```python
from build123d import *

# Parameters (mm, degrees)
SKETCH1_R           = 2.75
BOSS_EXTRUDE1_DEPTH = 6
FILLET1_R           = 3
SKETCH2_R           = 25.25
CUT_EXTRUDE1_DEPTH  = 3


with BuildPart() as part:
    # Sketch1 → Boss-Extrude1 (new body)
    with BuildSketch(Plane(origin=(0, 0, 0), x_dir=(1, 0, 0), z_dir=(0, 1, 0))):
        with BuildLine():
            Line((-57.629202667, 39.951533137), (-39.951533137, 57.629202667))
            Line((-39.951533137, 57.629202667), (-21.213203436, 38.890872965))
            ThreePointArc((-21.213203436, 38.890872965), (0, 30.104076401), (21.213203436, 38.890872965))
            Line((21.213203436, 38.890872965), (39.951533137, 57.629202667))
            Line((39.951533137, 57.629202667), (57.629202667, 39.951533137))
            Line((57.629202667, 39.951533137), (35.355339059, 17.67766953))
            Line((35.355339059, 17.67766953), (35.355339059, -17.67766953))
            Line((35.355339059, -17.67766953), (57.629202667, -39.951533137))
            Line((57.629202667, -39.951533137), (39.951533137, -57.629202667))
            Line((39.951533137, -57.629202667), (21.213203436, -38.890872965))
            ThreePointArc((21.213203436, -38.890872965), (0, -30.104076401), (-21.213203436, -38.890872965))
            Line((-21.213203436, -38.890872965), (-39.951533137, -57.629202667))
            Line((-39.951533137, -57.629202667), (-57.629202667, -39.951533137))
            Line((-57.629202667, -39.951533137), (-35.355339059, -17.67766953))
            Line((-35.355339059, -17.67766953), (-35.355339059, 17.67766953))
            Line((-35.355339059, 17.67766953), (-57.629202667, 39.951533137))
        make_face()
        with Locations(Location((-45.254833996, 45.254833996, 0), (0, 0, 270))):
            Circle(SKETCH1_R, mode=Mode.SUBTRACT)
        with Locations(Location((45.254833996, 45.254833996, 0), (0, 0, 270))):
            Circle(SKETCH1_R, mode=Mode.SUBTRACT)
        with Locations(Location((45.254833996, -45.254833996, 0), (0, 0, 270))):
            Circle(SKETCH1_R, mode=Mode.SUBTRACT)
        with Locations(Location((-45.254833996, -45.254833996, 0), (0, 0, 270))):
            Circle(SKETCH1_R, mode=Mode.SUBTRACT)
        with Locations(Location((-24.75, 24.75, 0), (0, 0, 270))):
            Circle(SKETCH1_R, mode=Mode.SUBTRACT)
        with Locations(Location((-24.75, -24.75, 0), (0, 0, 270))):
            Circle(SKETCH1_R, mode=Mode.SUBTRACT)
        with Locations(Location((24.75, -24.75, 0), (0, 0, 90))):
            Circle(SKETCH1_R, mode=Mode.SUBTRACT)
        with Locations(Location((24.75, 24.75, 0), (0, 0, 90))):
            Circle(SKETCH1_R, mode=Mode.SUBTRACT)
        with Locations(Location((-14.142135624, 14.142135624, 0), (0, 0, 270))):
            Circle(SKETCH1_R, mode=Mode.SUBTRACT)
        with Locations(Location((14.142135624, 14.142135624, 0), (0, 0, 270))):
            Circle(SKETCH1_R, mode=Mode.SUBTRACT)
        with Locations(Location((14.142135624, -14.142135624, 0), (0, 0, 270))):
            Circle(SKETCH1_R, mode=Mode.SUBTRACT)
        with Locations(Location((-14.142135624, -14.142135624, 0), (0, 0, 270))):
            Circle(SKETCH1_R, mode=Mode.SUBTRACT)
    extrude(amount=BOSS_EXTRUDE1_DEPTH)

    # Fillet1
    fillet1_edges = [part.edges().sort_by_distance(p)[0] for p in [
        (-57.629202667, 3, -39.951533137),
        (-39.951533137, 3, -57.629202667),
        (39.951533137, 3, -57.629202667),
        (57.629202667, 3, -39.951533137),
        (57.629202667, 3, 39.951533137),
        (39.951533137, 3, 57.629202667),
        (-39.951533137, 3, 57.629202667),
        (-57.629202667, 3, 39.951533137),
    ]]
    fillet(fillet1_edges, radius=FILLET1_R)

    # Sketch2 → Cut-Extrude1 (cut)
    with BuildSketch(Plane(origin=(0, 6, 0), x_dir=(1, 0, 0), z_dir=(0, 1, 0))):
        with Locations(Location((0, 0, 0), (0, 0, 270))):
            Circle(SKETCH2_R)
    extrude(amount=-CUT_EXTRUDE1_DEPTH, mode=Mode.SUBTRACT)


solid = part.part
```
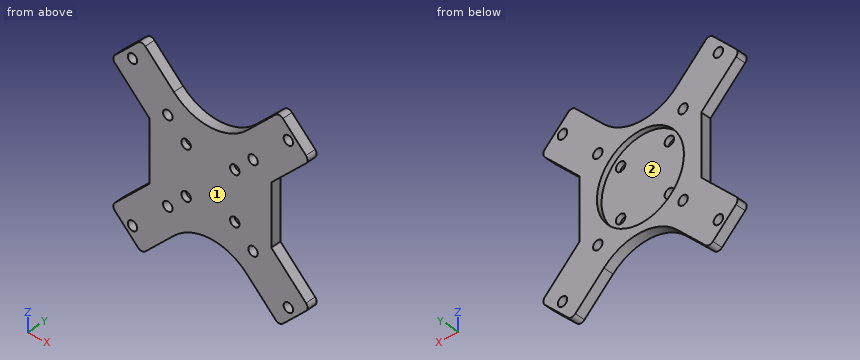
Check sheet for the modelled part. Datum: model origin and axes. Units: mm. Face numbers are marked on the shaded views. Coordinates: 2 decimals unless noted, no trailing zeros. Loops run counter-clockwise (first coordinate to the right, second up) from the corner with the lowest first, then second, coordinate; pieces in that order, holes last.
1) Sectioned sample at C-C (y = 4.15). Count the separate pieces of the cut face and the enclosed holes in it, and give its area (3 significant figures).
2) Sectioned sample at B-B (x = 0). Record the boundary of the cut face in (y, z).
3) Sectioned sample at D-D (z = -15). Record the boundary of the cut face in (x, y), and give its area (3 significant figures).
4) Release check for a two-part mould opening along X. For the marked faces 1 and 2 record: released by +X, released by -X, zero draft, split by the parting line, or undercut.
5) Material ranges on probe 1 along X at (y, z) = (4.95, -45); probe 2 along Z at (x, y) = (25.5, 4.5), recorded low to high.
6) Gauge pin test, flat ends, axial feed: pin 1 (1.8 mm diameter, centred on y = 1.5, z = 4, fed in from -X); pin 2 (4.5 mm diameter, centred on x = 14.14, z = 14.14, fed in from +Y); pin 3 (1.5 mm diameter, centred on x = -0.5, y = 1.5, fed in from +Z). Record the tip position at first contact, or that the pin passes through.
7) Sectioned sample at A-A (z = 0). Record the boundary of the cut face in (x, y).
Check sheet entries:
1. separate pieces: 1
1. enclosed holes: 9
1. area: 5,080 mm2
2. outline: (0, -30.1) - (6, -30.1) - (6, -25.25) - (3, -25.25) - (3, 25.25) - (6, 25.25) - (6, 30.1) - (0, 30.1) - close
3. outline: (-35.36, 0) - (-16.75, 0) - (-16.75, 3) - (-20.31, 3) - (-20.31, 6) - (-35.36, 6) - close; (-11.53, 0) - (11.53, 0) - (11.53, 3) - (-11.53, 3) - close; (16.75, 0) - (35.36, 0) - (35.36, 6) - (20.31, 6) - (20.31, 3) - (16.75, 3) - close
3. area: 271 mm2
4. face 1: zero draft
4. face 2: undercut
5. probe 1: x = -52.58 to -47.99, -42.52 to -27.32, 27.32 to 42.52, 47.99 to 52.58
5. probe 2: z = -43.18 to -27.4, -22.1 to 22.1, 27.4 to 43.18
6. pin 1: stops at x = -35.36
6. pin 2: passes through
6. pin 3: stops at z = 30.13
7. outline: (-35.36, 0) - (35.36, 0) - (35.36, 6) - (25.25, 6) - (25.25, 3) - (-25.25, 3) - (-25.25, 6) - (-35.36, 6) - close
